Can you work these out from the model? Positions are in its coordinate system, mm. Face numbers are marked on the shaded views. A direction names the side the tool comes from. Coordinates: 2 decimals unless noted, no trailing zeros. Order: outer loops, then holes, each group sorted by start corner. A loop starts at its lowest first (then second) coordinate and runs counter-clockwise, first axis right, second up. Notation, with made-up numbers: (-2.5, -30.5) - (15.5, -30.5) arc R33 cw to (15.5, 8.5) - close; hole circle Ø2 at (-35, 33.25). An arc over 180 degrees is marked (long way). Return JSON: item names as keys, results as strings. Group by question number.
1) Imagine slicing it at C-C (y = 3.25). Write out the boundary of the cut face in (x, z) (3 decimals), and give its area (3 significant figures).
2) If we mould it in two halves opening along Y, with no side actions, what happens to the marked faces 4, 5 and 6? For each: pulls with the +Y half, pulls with the -Y half, needs draft (parallel to the pull), parting line crosses it, or undercut.
3) Imagine slicing it at D-D (z = 4.75). Write out the boundary of the cut face in (x, y), and give its area (3 significant figures).
4) Imagine slicing it at A-A (y = 0). Write out the boundary of the cut face in (x, z) (3 decimals), and give its area (3 significant figures).
5) For pin 1 Ø6 at (x, y) = (0.5, -0.5) entering from -Z (3 decimals); pin 2 Ø2.5 at (x, z) = (0, 6.35) entering from +Y; pin 3 Ø3 at (x, z) = (-2, 4) entering from -Y; pin 4 Ø1.5 at (y, z) = (2.5, 0) entering from -X, each with a flat end and sliding along its axis, tell me the tip position at first contact or that it passes through.
6) Imagine slicing it at B-B (x = 0). Write out the boundary of the cut face in (y, z) (3 decimals), and give its area (3 significant figures).
7) If I drill on line 1 along Y through (x, z) = (0, 1.5); line 2 along Z through (x, y) = (0, 4.2) (3 decimals); line 3 along Y through (x, z) = (4.5, 2.75), over which ranges is the centre line in solid material (lowest first)?
8) Which directions (+Z, -Z, +X, -X, +Y, -Y) give clear straight access to the entire face, cutting with the end or side of a thin tool? Please do the marked faces 1, 2 and 3.
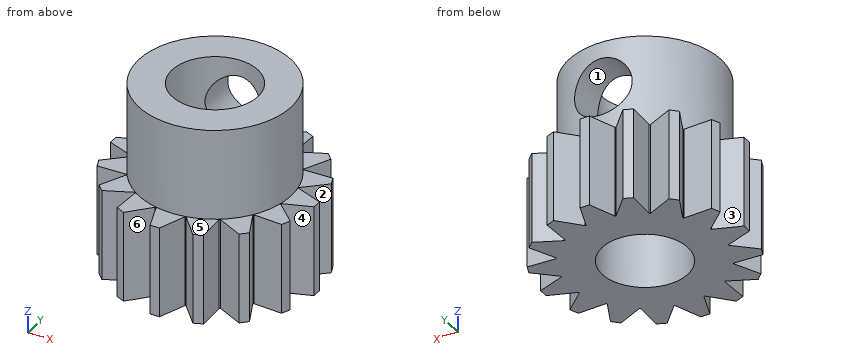
```python
from build123d import *

# Parameters (mm, degrees)
BOSS_EXTRUDE1_DEPTH              = 6.35
SKETCH2_W                        = 5.3213
SKETCH2_H                        = 6.35
F_12_CLEARANCE_HOLE1_D           = 6
F_21_0_159_DIAMETER_HOLE1_REACH  = 19.23
F_21_0_159_DIAMETER_HOLE1_BORE_R = 2.0193


with BuildPart() as part:
    # Sketch1 → Boss-Extrude1 (new body)
    with BuildSketch(Plane.XY.offset(3.175)):
        with BuildLine():
            Line((2.945181061, 4.475719374), (3.032230323, 6.469475256))
            Line((3.032230323, 6.469475256), (2.430499075, 6.7187205))
            Line((2.430499075, 6.7187205), (1.082253901, 5.247369083))
            ThreePointArc((1.082253901, 5.247369083), (1.045257317, 5.254863741), (1.008208849, 5.262097559))
            Line((1.008208849, 5.262097559), (0.325654523, 7.137400133))
            Line((0.325654523, 7.137400133), (-0.325654702, 7.137400133))
            Line((-0.325654702, 7.137400133), (-1.008209026, 5.262097541))
            ThreePointArc((-1.008209026, 5.262097541), (-1.045257435, 5.254863734), (-1.082253959, 5.247369087))
            Line((-1.082253959, 5.247369087), (-2.43049913, 6.718720502))
            Line((-2.43049913, 6.718720502), (-3.03223038, 6.469475257))
            Line((-3.03223038, 6.469475257), (-2.945181121, 4.475719388))
            ThreePointArc((-2.945181121, 4.475719388), (-2.976641184, 4.454858374), (-3.007953492, 4.433776229))
            Line((-3.007953492, 4.433776229), (-4.816631407, 5.277176573))
            Line((-4.816631407, 5.277176573), (-5.277176625, 4.816631474))
            Line((-5.277176625, 4.816631474), (-4.433776215, 3.007953457))
            ThreePointArc((-4.433776215, 3.007953457), (-4.454858319, 2.976641205), (-4.475719295, 2.945181199))
            Line((-4.475719295, 2.945181199), (-6.469475174, 3.032230463))
            Line((-6.469475174, 3.032230463), (-6.718720419, 2.430499213))
            Line((-6.718720419, 2.430499213), (-5.247368979, 1.082254018))
            ThreePointArc((-5.247368979, 1.082254018), (-5.254863646, 1.045257392), (-5.26209747, 1.008208882))
            Line((-5.26209747, 1.008208882), (-7.137400023, 0.325654551))
            Line((-7.137400023, 0.325654551), (-7.137400023, -0.325654674))
            Line((-7.137400023, -0.325654674), (-5.262097383, -1.008209015))
            ThreePointArc((-5.262097383, -1.008209015), (-5.254863591, -1.045257342), (-5.24736896, -1.082253784))
            Line((-5.24736896, -1.082253784), (-6.71872042, -2.430498991))
            Line((-6.71872042, -2.430498991), (-6.469475175, -3.032230242))
            Line((-6.469475175, -3.032230242), (-4.475719227, -2.945180979))
            ThreePointArc((-4.475719227, -2.945180979), (-4.454858236, -2.976641007), (-4.433776114, -3.007953281))
            Line((-4.433776114, -3.007953281), (-5.277176492, -4.816631269))
            Line((-5.277176492, -4.816631269), (-4.816631393, -5.277176487))
            Line((-4.816631393, -5.277176487), (-3.007953296, -4.433776039))
            ThreePointArc((-3.007953296, -4.433776039), (-2.976641082, -4.454858118), (-2.945181114, -4.475719068))
            Line((-2.945181114, -4.475719068), (-3.03223038, -6.469475037))
            Line((-3.03223038, -6.469475037), (-2.43049913, -6.718720282))
            Line((-2.43049913, -6.718720282), (-1.082253881, -5.24736878))
            ThreePointArc((-1.082253881, -5.24736878), (-1.045257351, -5.254863427), (-1.008208937, -5.262097234))
            Line((-1.008208937, -5.262097234), (-0.325654579, -7.137399864))
            Line((-0.325654579, -7.137399864), (0.325654646, -7.137399864))
            Line((0.325654646, -7.137399864), (1.008209007, -5.262097205))
            ThreePointArc((1.008209007, -5.262097205), (1.045257357, -5.25486341), (1.082253822, -5.247368775))
            Line((1.082253822, -5.247368775), (2.430499075, -6.718720281))
            Line((2.430499075, -6.718720281), (3.032230325, -6.469475036))
            Line((3.032230325, -6.469475036), (2.945181058, -4.475719052))
            ThreePointArc((2.945181058, -4.475719052), (2.976641071, -4.454858071), (3.00795333, -4.433775961))
            Line((3.00795333, -4.433775961), (4.816631352, -5.277176352))
            Line((4.816631352, -5.277176352), (5.27717657, -4.816631253))
            Line((5.27717657, -4.816631253), (4.433776119, -3.007953154))
            ThreePointArc((4.433776119, -3.007953154), (4.454858198, -2.976640942), (4.475719148, -2.945180976))
            Line((4.475719148, -2.945180976), (6.469475118, -3.032230242))
            Line((6.469475118, -3.032230242), (6.718720363, -2.430498991))
            Line((6.718720363, -2.430498991), (5.247368883, -1.082253764))
            ThreePointArc((5.247368883, -1.082253764), (5.254863535, -1.045257218), (5.262097345, -1.008208788))
            Line((5.262097345, -1.008208788), (7.137399945, -0.32565444))
            Line((7.137399945, -0.32565444), (7.137399945, 0.325654785))
            Line((7.137399945, 0.325654785), (5.262097343, 1.008209124))
            ThreePointArc((5.262097343, 1.008209124), (5.254863542, 1.045257505), (5.247368901, 1.082254002))
            Line((5.247368901, 1.082254002), (6.718720362, 2.430499213))
            Line((6.718720362, 2.430499213), (6.469475118, 3.032230461))
            Line((6.469475118, 3.032230461), (4.475719213, 2.9451812))
            ThreePointArc((4.475719213, 2.9451812), (4.45485821, 2.976641248), (4.433776076, 3.007953541))
            Line((4.433776076, 3.007953541), (5.277176433, 4.81663149))
            Line((5.277176433, 4.81663149), (4.816631336, 5.277176706))
            Line((4.816631336, 5.277176706), (3.007953315, 4.433776294))
            ThreePointArc((3.007953315, 4.433776294), (2.976641065, 4.454858399), (2.945181061, 4.475719374))
        make_face()
    extrude(amount=-BOSS_EXTRUDE1_DEPTH)

    # Sketch2 → Revolve1 (revolve)
    with BuildSketch(Plane.XZ, mode=Mode.PRIVATE) as revolve1_sk:
        with Locations((2.66065, 6.35)):
            Rectangle(SKETCH2_W, SKETCH2_H)
    revolve(revolve1_sk.sketch.rotate(Axis((0, 0, 9.525), (0, 0, -1)), 180), axis=Axis((0, 0, 9.525), (0, 0, -1)))

    # #12 Clearance Hole1 (through all)
    with Locations(Plane.XY.offset(9.525)):
        with Locations((0, 0)):
            Hole(F_12_CLEARANCE_HOLE1_D / 2)

    # #21 (0.159) Diameter Hole1 bore (on position points) → #21 (0.159) Diameter Hole1 (cut, up to next)
    with BuildSketch(Plane(origin=(0, 5.3213, 6.35), x_dir=(1, 0, 0), z_dir=(0, 1, 0)), mode=Mode.PRIVATE) as f_21_0_159_diameter_hole1_sk1:
        Circle(F_21_0_159_DIAMETER_HOLE1_BORE_R)
    f_21_0_159_diameter_hole1_tool1 = extrude(f_21_0_159_diameter_hole1_sk1.sketch, amount=-F_21_0_159_DIAMETER_HOLE1_REACH, mode=Mode.PRIVATE) & part.part
    add(f_21_0_159_diameter_hole1_tool1.solids().sort_by_distance((0, 5.3213, 6.35))[0], mode=Mode.SUBTRACT)


solid = part.part
```
Calculated:
{
 "1": {"outline": "(-4.547, -3.175) - (4.547, -3.175) - (4.547, 3.175) - (4.214, 3.175) - (4.214, 9.525) - (-4.214, 9.525) - (-4.214, 3.175) - (-4.547, 3.175) - close; hole circle Ø4.039 at (0, 6.35)", "area": "98.4 mm2"},
 "2": {"face 4": "undercut", "face 5": "needs draft", "face 6": "pulls with the -Y half"},
 "3": {"outline": "(-1.23, 2.74) - (-1.23, 5.18) arc R5.32 ccw (long way) to (1.23, 5.18) - (1.23, 2.74) arc R3 cw (long way) to start", "area": "54.9 mm2"},
 "4": {"outline": "(-7.137, -3.175) - (-3, -3.175) - (-3, 9.525) - (-5.321, 9.525) - (-5.321, 3.175) - (-7.137, 3.175) - close; (3, -3.175) - (7.137, -3.175) - (7.137, 3.175) - (5.321, 3.175) - (5.321, 9.525) - (3, 9.525) - close", "area": "82.0 mm2"},
 "5": {"pin 1": "z = -3.175", "pin 2": "y = -2.73", "pin 3": "y = -6.72", "pin 4": "x = -6.72"},
 "6": {"outline": "(-7.137, -3.175) - (-3, -3.175) - (-3, 9.525) - (-5.321, 9.525) - (-5.321, 3.175) - (-7.137, 3.175) - close; (3, -3.175) - (7.137, -3.175) - (7.137, 3.175) - (5.321, 3.175) - (5.321, 4.331) - (3, 4.331) - close; (3, 8.369) - (5.321, 8.369) - (5.321, 9.525) - (3, 9.525) - close", "area": "72.7 mm2"},
 "7": {"line 1": "-7.14 to -3, 3 to 7.14", "line 2": "-3.175 to 4.331, 8.369 to 9.525", "line 3": "-5.13 to -3.15, -2.95 to 2.95, 3.15 to 5.13"},
 "8": {"face 1": "+Y", "face 2": "+Z, -Z, +X", "face 3": "+Z, -Z, -X"}
}
